Check sheet for the modelled part. Datum: model origin and axes. Units: mm. A direction names the side the tool comes from. Give positions to 0.01 mm unless a question says otherwise; leave off trailing zeros. Write each loop counter-clockwise with the first axis right and the second up, starting at its lowest first coordinate (ties: lowest second). Pieces come first, ordered by that corner, then holes. Notation, with made-up numbers: M 72.5,83.25 L 109.5,83.25 A11 cw 109.5,100.25 Z; hole C 34,-2 d10. An arc over 180 degrees is marked long. Write item = value, one per line. Start each with the question number.
1) Mould release check, pull along X, two halves, no side actions. Record for faces 3 (the cylindrical face through (-3.955, -2.465, -5.158)), 4 (the flat face through (-1, -20, -11)), 5 (the flat face through (-65, -10, 1)): released by +X, released by -X, zero draft, split by the parting line, or undercut.
2) Scan lines: line 1 along X through (y, z) = (-16, 0); line 2 along X through (y, z) = (-2.1, 0); line 3 along X through (y, z) = (-8, -44). Record each from-to range of solid material in increasing order. Write a range as [from, to].
3) Cross-section at A-A, the plane z = 0. Record the cut outline in (x, y), plus the area to 3 significant figures.
4) Cross-section at B-B, the plane x = 0. Record the cut outline in (y, z).
5) Go/stop test with a flat-tipped pin: pin 1 (8.5 mm diameter, centred on x = 0, z = 0, fed in from -Y). Record where the tip stops, or that it passes through.
6) Access from +Z, -Z, +X, -X, +Y, -Y to the whole of each face (thin tool, end or side, straight path). Record for faces 1 (the cylindrical face through (-63.57, -10.14, 47)), 2 (the flat face through (5, -5, 2)).
```python
from build123d import *

# Parameters (mm, degrees)
SKETCH1_W           = 130
SKETCH1_H           = 97
BOSS_EXTRUDE1_DEPTH = 20
SKETCH2_R           = 5.2
CUT_EXTRUDE1_DEPTH  = 84.529934754
SKETCH3_R           = 6.5
CUT_EXTRUDE2_DEPTH  = 5
FILLET1_R           = 5


with BuildPart() as part:
    # Sketch1 → Boss-Extrude1 (new body)
    with BuildSketch(Plane(origin=(0, 0, 0), x_dir=(1, 0, 0), z_dir=(0, 1, 0))):
        Rectangle(SKETCH1_W, SKETCH1_H)
    extrude(amount=-BOSS_EXTRUDE1_DEPTH)

    # Sketch2 → Cut-Extrude1 (cut, through all)
    with BuildSketch(Plane(origin=(0, 0, 0), x_dir=(1, 0, 0), z_dir=(0, 1, 0))):
        with Locations(Location((0, 0, 0), (0, 0, 270))):
            Circle(SKETCH2_R)
    extrude(amount=-CUT_EXTRUDE1_DEPTH, mode=Mode.SUBTRACT)

    # Sketch3 → Cut-Extrude2 (cut)
    with BuildSketch(Plane(origin=(0, 0, 0), x_dir=(1, 0, 0), z_dir=(0, 1, 0))):
        with Locations(Location((0, 0, 0), (0, 0, 270))):
            Circle(SKETCH3_R)
    extrude(amount=-CUT_EXTRUDE2_DEPTH, mode=Mode.SUBTRACT)

    # Fillet1
    fillet1_edges = [part.edges().sort_by_distance(p)[0] for p in [
        (65, -10, 48.5),
        (-65, -10, 48.5),
        (-65, -10, -48.5),
        (65, -10, -48.5),
    ]]
    fillet(fillet1_edges, radius=FILLET1_R)


solid = part.part
```
Reply:
q1.face_3 = undercut
q1.face_4 = zero draft
q1.face_5 = released by -X
q2.line_1 = [-65, -5.2], [5.2, 65]
q2.line_2 = [-65, -6.5], [6.5, 65]
q2.line_3 = [-64.97, 64.97]
q3.outline = M -65,-20 L -5.2,-20 L -5.2,-5 L -6.5,-5 L -6.5,0 L -65,0 Z; M 5.2,-20 L 65,-20 L 65,0 L 6.5,0 L 6.5,-5 L 5.2,-5 Z
q3.area = 2,380 mm2
q4.outline = M -20,-48.5 L 0,-48.5 L 0,-6.5 L -5,-6.5 L -5,-5.2 L -20,-5.2 Z; M -20,5.2 L -5,5.2 L -5,6.5 L 0,6.5 L 0,48.5 L -20,48.5 Z
q5.pin_1 = through
q6.face_1 = +Z, -X, +Y, -Y
q6.face_2 = +Y
